```python
from build123d import *

# Parameters (mm, degrees)
F1_DEPTH  = 28
F0_W      = 34
F0_H      = 70
F0_R      = 2
F0_H_2    = 5
F2_DEPTH  = 5
F3_DEPTH  = 12
F0_W_2    = 5
F4_DEPTH  = 5
F5_DEPTH  = 28
F6_DEPTH  = 12
F7_W      = 5
F7_H      = 80
F8_DEPTH  = 15
F9_W      = 5
F9_H      = 9
F10_DEPTH = 24.501
F11_W     = 3
F11_H     = 8
F12_DEPTH = 80.001
F13_DEPTH = 24.501


with BuildPart() as f1:
    # F0 (on Top) → F1 (new body)
    with BuildSketch(Plane.XY):
        Polygon((-17, 37.5), (-22, 37.5), (-22, -37.5), (-17, -37.5), (-17, -32.5), align=None)
        Polygon((22, 37.5), (17, 37.5), (17, -32.5), (17, -37.5), (22, -37.5), align=None)
    extrude(amount=F1_DEPTH)

    # F0 (on Top) → F2 (join)
    with BuildSketch(Plane.XY):
        Polygon((-17, 37.5), (-22, 37.5), (-22, -37.5), (-17, -37.5), (-17, -32.5), align=None)
        with Locations((0, 2.5)):
            Rectangle(F0_W, F0_H)
        with Locations((-13, -13)):
            Circle(F0_R, mode=Mode.SUBTRACT)
        with Locations((13, -13)):
            Circle(F0_R, mode=Mode.SUBTRACT)
        with Locations((-13, 13)):
            Circle(F0_R, mode=Mode.SUBTRACT)
        with Locations((13, 13)):
            Circle(F0_R, mode=Mode.SUBTRACT)
        Polygon((22, 37.5), (17, 37.5), (17, -32.5), (17, -37.5), (22, -37.5), align=None)
        with Locations((0, -35)):
            Rectangle(F0_W, F0_H_2)
    extrude(amount=-F2_DEPTH)

    # F0 (on Top) → F3 (join)
    with BuildSketch(Plane.XY):
        with Locations((0, -35)):
            Rectangle(F0_W, F0_H_2)
    extrude(amount=F3_DEPTH)

    # F0 (on Top) → F4 (join, through all)
    with BuildSketch(Plane.XY):
        with Locations((19.5, 40)):
            Rectangle(F0_W_2, F0_H_2)
        with Locations((0, 40)):
            Rectangle(F0_W, F0_H_2)
        with Locations((-19.5, 40)):
            Rectangle(F0_W_2, F0_H_2)
    extrude(amount=-F4_DEPTH)

    # F0 (on Top) → F5 (join, through all)
    with BuildSketch(Plane.XY):
        with Locations((19.5, 40)):
            Rectangle(F0_W_2, F0_H_2)
        with Locations((-19.5, 40)):
            Rectangle(F0_W_2, F0_H_2)
    extrude(amount=F5_DEPTH)

    # F0 (on Top) → F6 (join)
    with BuildSketch(Plane.XY):
        with Locations((0, 40)):
            Rectangle(F0_W, F0_H_2)
    extrude(amount=F6_DEPTH)

    # F7 (on face) → F8 (join)
    with BuildSketch(Plane(origin=(0, 0, -5), x_dir=(1, 0, 0), z_dir=(0, 0, -1))):
        with Locations((0, -2.5)):
            Rectangle(F7_W, F7_H)
    extrude(amount=F8_DEPTH)

    # F9 (on face) → F10 (cut, through all)
    with BuildSketch(Plane.YZ.offset(2.5)):
        with Locations((-30, -10.5)):
            Rectangle(F9_W, F9_H)
    extrude(amount=-F10_DEPTH, mode=Mode.SUBTRACT)

    # F11 (on face) → F12 (cut, through all)
    with BuildSketch(Plane.XZ.offset(37.5)):
        with Locations((-4, 4)):
            Rectangle(F11_W, F11_H)
        with Locations((4, 4)):
            Rectangle(F11_W, F11_H)
    extrude(amount=-F12_DEPTH, mode=Mode.SUBTRACT)

    # F9 (on face) → F13 (cut, through all)
    with BuildSketch(Plane.YZ.offset(2.5)):
        with Locations((35, -10.5)):
            Rectangle(F9_W, F9_H)
    extrude(amount=-F13_DEPTH, mode=Mode.SUBTRACT)


solid = f1.part
```
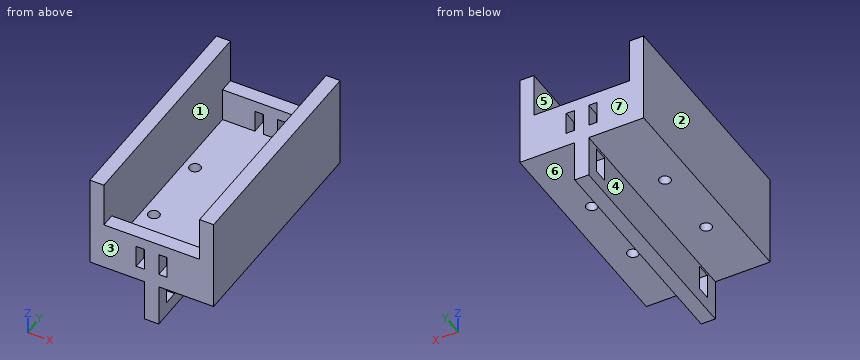
Source: CAD feature listing. Evaluate the final solid. Frame: model axes, mm. Face numbers are marked on the shaded views. A direction names the side the tool comes from. Round coordinates to 2 decimals unless told otherwise and drop trailing zeros. Loops run counter-clockwise (first coordinate to the right, second up) from the corner with the lowest first, then second, coordinate; pieces in that order, holes last.
(1) Section query A-A (y = -30). Output: boundary loops of the cut face in (x, z).
From the geometry:
outline: (-22, -5) - (-2.5, -5) - (-2.5, -6) - (2.5, -6) - (2.5, -5) - (22, -5) - (22, 28) - (17, 28) - (17, 0) - (-17, 0) - (-17, 28) - (-22, 28) - close; (-2.5, -20) - (2.5, -20) - (2.5, -15) - (-2.5, -15) - close
(2) Access query for the marked faces 4, 5, 6 and 7. Directions: +Z, -Z, +X, -X, +Y, -Y. A direction counts if a zero-diameter tool reaches every point of the face in a straight line with its end or side. Return the directions, or none.
From the geometry:
face 4: -Z, -X, +Y, -Y
face 5: +Z
face 6: -Z, +X, +Y, -Y
face 7: +Z, -Z, +X, -X, +Y
(3) Material intervals for probe 1 along Y at (x, z) = (13, -1); probe 2 along Y at (x, z) = (6, 7); probe 3 along X at (y, z) = (29.5, 4.5), sorted ascending.
From the geometry:
probe 1: y = -37.5 to -15, -11 to 11, 15 to 42.5
probe 2: y = -37.5 to -32.5, 37.5 to 42.5
probe 3: x = -22 to -17, 17 to 22
(4) Section query D-D (y = 13). Output: boundary loops of the cut face in (x, z), and give its area (3 significant figures).
From the geometry:
outline: (-22, -5) - (-15, -5) - (-15, 0) - (-17, 0) - (-17, 28) - (-22, 28) - close; (-11, -5) - (-2.5, -5) - (-2.5, -20) - (2.5, -20) - (2.5, -5) - (11, -5) - (11, 0) - (-11, 0) - close; (15, -5) - (22, -5) - (22, 28) - (17, 28) - (17, 0) - (15, 0) - close
area: 535 mm2
(5) Section query C-C (x = 13). Output: boundary loops of the cut face in (y, z).
From the geometry:
outline: (-37.5, -5) - (-15, -5) - (-15, 0) - (-32.5, 0) - (-32.5, 12) - (-37.5, 12) - close; (-11, -5) - (11, -5) - (11, 0) - (-11, 0) - close; (15, -5) - (42.5, -5) - (42.5, 12) - (37.5, 12) - (37.5, 0) - (15, 0) - close
(6) Pull-direction query (Y, two-part tool) for the marked faces 1, 2 and 3; classes: +Y half, -Y half, draft (parallel to the pull), parting line (faces both ways), or undercut.
From the geometry:
face 1: undercut
face 2: draft
face 3: -Y half
(7) Section query B-B (z = 20). Output: boundary loops of the cut face in (x, y).
From the geometry:
outline: (-22, -37.5) - (-17, -37.5) - (-17, 42.5) - (-22, 42.5) - close; (17, -37.5) - (22, -37.5) - (22, 42.5) - (17, 42.5) - close
(8) Contact query for flat-ended pins moving along their axis: pin 1 Ø6.5 at (x, y) = (13, -13) entering from +Z; pin 2 Ø6 at (x, y) = (-13, -9.5) entering from -Z; pin 3 Ø3 at (y, z) = (15, -7.5) entering from +X. Output: stop coordinate, or through.
From the geometry:
pin 1: stops at z = 0
pin 2: stops at z = -5
pin 3: stops at x = 2.5
